Source: three-view drawing plus pictorial views. Frame: mm from the lowest corner of the part. Round coordinates to 2 decimals unless told otherwise and drop trailing zeros. Order: outer loops, then holes, each group sorted by start corner. A loop starts at its lowest first (then second) coordinate and runs counter-clockwise, first axis right, second up. Notation, with made-up numbers: M 28,64 L 39,64 A4 ccw 39,68 Z; hole C 41.5,8.5 d8. An arc over 180 degrees is marked long. Return JSON: item names as keys, results as strings. Group by question number.
Q1. Cut plane A-A on y = 72.5. Output: boundary loops of the cut face in (x, z), and give its area (4 significant figures).
Q2. Cut plane C-C on z = 9. Output: boundary loops of the cut face in (x, y) (1 decimal), and give its area (3 significant figures).
Q3. Mould query, pull axis Y, two halves, no side actions, for the marked faces 1, 2 and 3. Classes: released by +Y, released by -Y, zero draft, split by the parting line, or undercut.
Q4. Ray query, probe 1 along X at (y, z) = (68.5, 23) (1 decimal); probe 2 along Y at (x, z) = (84.5, 26.5); probe 3 along X at (y, z) = (45, 45.5). Return the intervals inside material, ascending.
Q5. Cut plane B-B on x = 72. Output: boundary loops of the cut face in (y, z) (1 decimal).
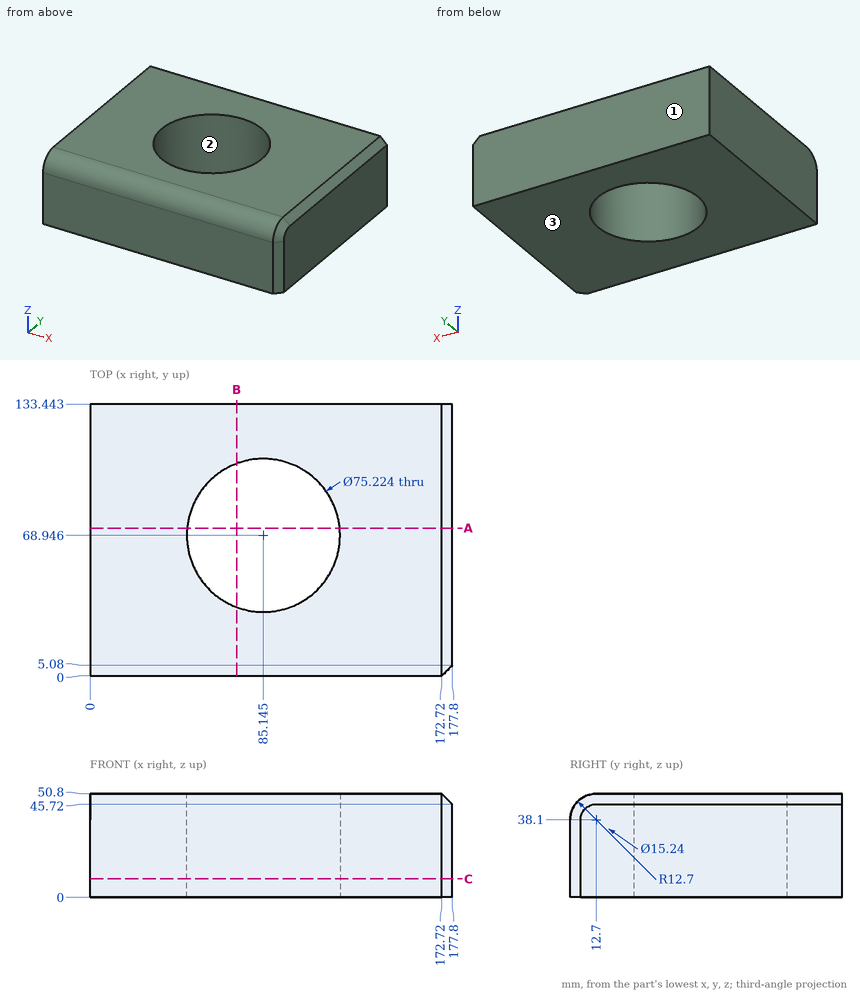
Result sheet:
{
 "1": {"outline": "M 0,0 L 47.7,0 L 47.7,50.8 L 0,50.8 Z; M 122.59,0 L 177.8,0 L 177.8,45.72 L 172.72,50.8 L 122.59,50.8 Z", "area": "5,215 mm²"},
 "2": {"outline": "M 0,0 L 172.7,0 L 177.8,5.1 L 177.8,133.4 L 0,133.4 Z; hole C 85.1,68.9 d75.2", "area": "19,300 mm²"},
 "3": {"face 1": "released by +Y", "face 2": "undercut", "face 3": "zero draft"},
 "4": {"probe 1": "x = 0 to 47.5, 122.8 to 177.8", "probe 2": "y = 0 to 31.34, 106.55 to 133.44", "probe 3": "x = 0 to 56.14, 114.15 to 177.8"},
 "5": {"outline": "M 0,0 L 33.7,0 L 33.7,50.8 L 12.7,50.8 A12.7 ccw 0,38.1 Z; M 104.2,0 L 133.4,0 L 133.4,50.8 L 104.2,50.8 Z"}
}
